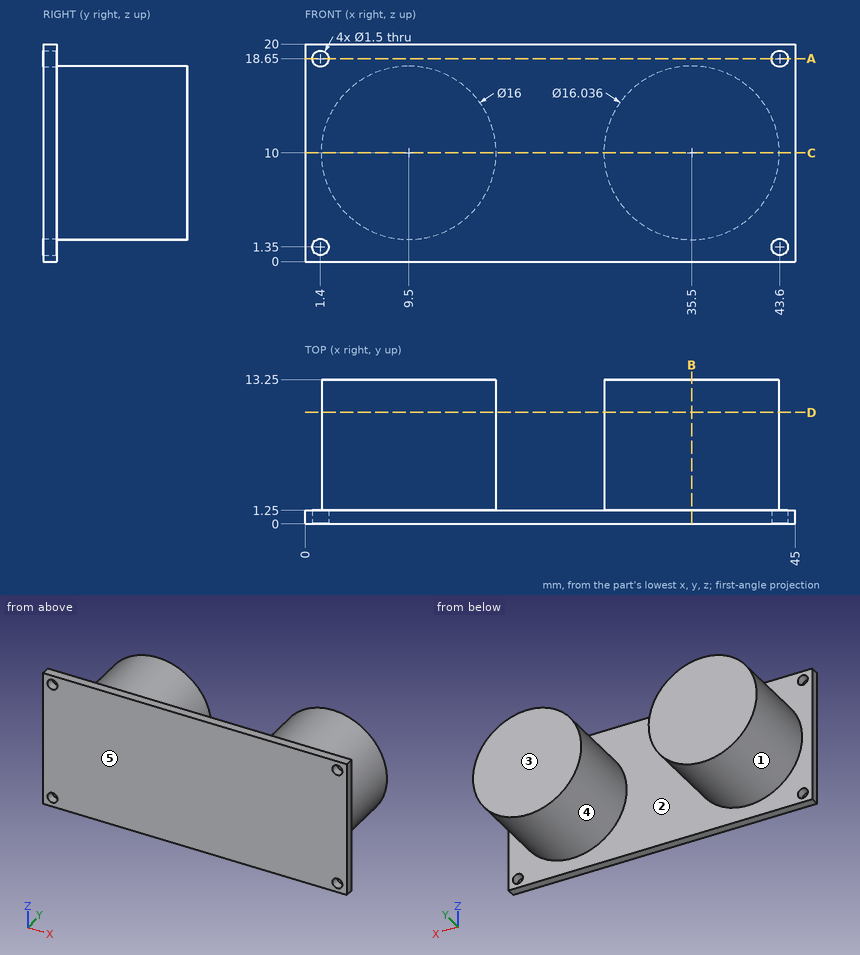
Could you check a few things on this drawing? It's one solid part, dimensions in mm from its lowest x, y, z. A direction names the side the tool comes from. Coordinates: 2 decimals unless noted, no trailing zeros. Loops run counter-clockwise (first coordinate to the right, second up) from the corner with the lowest first, then second, coordinate; pieces in that order, holes last.
1. We'd pull the mould along X, two halves only. Please class the marked faces 1, 2 and 3: released by +X, released by -X, zero draft, split by the parting line, or undercut.
2. Imagine slicing it at C-C (z = 10). Please give me the cut outline in (x, y).
3. Imagine slicing it at A-A (z = 18.65). Please give me the cut outline in (x, y), and give its area (3 significant figures).
4. For the marked faces 4 and 5, which set-ups out of +Z, -Z, +X, -X, +Y, -Y let a thin tool reach every point of the face, with its end or its side?
5. Imagine slicing it at D-D (y = 10.25). Please give me the cut outline in (x, z), and give its area (3 significant figures).
6. I need wall thicknesses on L1, parallel to X at y = 0.55, z = 18.65; L2, parallel to Z at x = 43.6, y = 0.4; L3, parallel to Y at x = 4, z = 18.25. Which ranges of each line are inside material? Lowest first, please.
7. Imagine slicing it at B-B (x = 35.5). Please give me the cut outline in (y, z), and give its area (3 significant figures).
8. For P1, Ø10, axis at x = 23, z = 15.5, coming from the +Y side; P2, Ø3, axis at y = 6, z = 8, coming from the +X side; P3, Ø0.9, axis at x = 1.4, z = 18.65, coming from the -Y side; P4, Ø1.5, axis at y = 3.5, z = 13, coming from the +X side, each with a flat end and sliding along its axis, tell me the tip position at first contact or that it passes through.
Computed values:
1. face 1: undercut
1. face 2: undercut
1. face 3: zero draft
2. outline: (0, 0) - (45, 0) - (45, 1.25) - (43.52, 1.25) - (43.52, 13.25) - (27.48, 13.25) - (27.48, 1.25) - (17.5, 1.25) - (17.5, 13.25) - (1.5, 13.25) - (1.5, 1.25) - (0, 1.25) - close
3. outline: (0, 0) - (0.65, 0) - (0.65, 1.25) - (0, 1.25) - close; (2.15, 0) - (42.85, 0) - (42.85, 1.25) - (2.15, 1.25) - close; (44.35, 0) - (45, 0) - (45, 1.25) - (44.35, 1.25) - close
3. area: 52.5 mm2
4. face 4: +Y
4. face 5: +Z, -Z, +X, -X, -Y
5. outline: circle Ø16 at (9.5, 10); circle Ø16.04 at (35.5, 10)
5. area: 403 mm2
6. L1: x = 0 to 0.65, 2.15 to 42.85, 44.35 to 45
6. L2: z = 0 to 0.6, 2.1 to 17.9, 19.4 to 20
6. L3: y = 0 to 1.25
7. outline: (0, 0) - (1.25, 0) - (1.25, 1.98) - (13.25, 1.98) - (13.25, 18.02) - (1.25, 18.02) - (1.25, 20) - (0, 20) - close
7. area: 217 mm2
8. P1: stops at y = 1.25
8. P2: stops at x = 43.5
8. P3: passes through
8. P4: stops at x = 43.2
